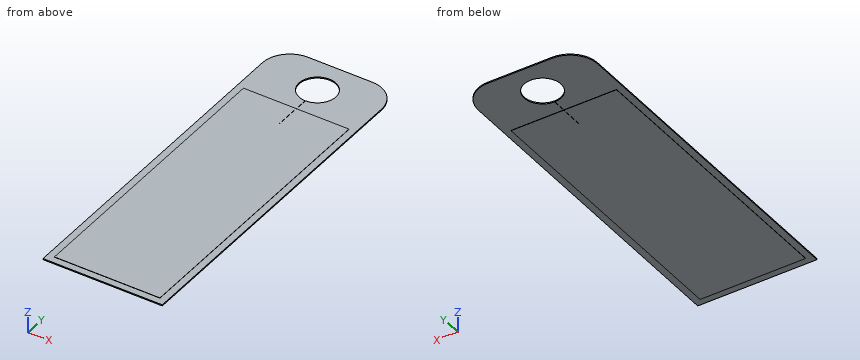
```python
from build123d import *

# Parameters (mm, degrees)
SKETCH2_R                = 8
BOSS_EXTRUDE1_DEPTH      = 0.5
BOSS_EXTRUDE2_DEPTH      = 0.1
BOSS_EXTRUDE2_DEPTH_BACK = 0.6
SKETCH4_W                = 46
SKETCH4_H                = 125
CUT_EXTRUDE1_DEPTH       = 145.361906333
CUT_EXTRUDE1_DEPTH_BACK  = 145.361906333
SKETCH5_W                = 0.1
SKETCH5_H                = 25


with BuildPart() as part:
    # Sketch2 → Boss-Extrude1 (new body)
    with BuildSketch(Plane.XY):
        with BuildLine():
            Line((-14, 15), (14, 15))
            ThreePointArc((14, 15), (22.485281374, 11.485281374), (26, 3))
            Line((26, 3), (26, -142))
            Line((26, -142), (-26, -142))
            Line((-26, -142), (-26, 3))
            ThreePointArc((-26, 3), (-22.485281374, 11.485281374), (-14, 15))
        make_face()
        Circle(SKETCH2_R, mode=Mode.SUBTRACT)
    extrude(amount=BOSS_EXTRUDE1_DEPTH)

    # Sketch4 → Boss-Extrude2 (add, two sides: drawn at the far end of the back side and taken through both)
    with BuildSketch(Plane.XY.offset(0.5).offset(-BOSS_EXTRUDE2_DEPTH_BACK)):
        with Locations((0, -76.5)):
            Rectangle(SKETCH4_W, SKETCH4_H)
    extrude(amount=BOSS_EXTRUDE2_DEPTH + BOSS_EXTRUDE2_DEPTH_BACK)

    # Sketch5 → Cut-Extrude1 (cut, two sides: drawn at the far end of the back side and taken through both)
    with BuildSketch(Plane.XY.offset(0.5).offset(-CUT_EXTRUDE1_DEPTH_BACK)):
        with Locations((0, -12.5)):
            Rectangle(SKETCH5_W, SKETCH5_H)
    extrude(amount=CUT_EXTRUDE1_DEPTH + CUT_EXTRUDE1_DEPTH_BACK, mode=Mode.SUBTRACT)


solid = part.part
```
Build history of the part. All positions in model axes, mm. Coordinates: 2 decimals unless noted, no trailing zeros. Write each loop counter-clockwise with the first axis right and the second up, starting at its lowest first coordinate (ties: lowest second). Pieces come first, ordered by that corner, then holes.
1. Band-saw the part on C-C, the plane x = 16. Give the cut face in (y, z).
Answer block:
outline: (-142, 0) - (-139, 0) - (-139, -0.1) - (-14, -0.1) - (-14, 0) - (14.83, 0) - (14.83, 0.5) - (-14, 0.5) - (-14, 0.6) - (-139, 0.6) - (-139, 0.5) - (-142, 0.5) - close
2. Band-saw the part on B-B, the plane y = -95. Give the cut face in (x, z), and give its area (3 significant figures).
Answer block:
outline: (-26, 0) - (-23, 0) - (-23, -0.1) - (23, -0.1) - (23, 0) - (26, 0) - (26, 0.5) - (23, 0.5) - (23, 0.6) - (-23, 0.6) - (-23, 0.5) - (-26, 0.5) - close
area: 35.2 mm2
3. Band-saw the part on A-A, the plane x = -3. Give the cut face in (y, z), and give its area (3 significant figures).
Answer block:
outline: (-142, 0) - (-139, 0) - (-139, -0.1) - (-14, -0.1) - (-14, 0) - (-7.42, 0) - (-7.42, 0.5) - (-14, 0.5) - (-14, 0.6) - (-139, 0.6) - (-139, 0.5) - (-142, 0.5) - close; (7.42, 0) - (15, 0) - (15, 0.5) - (7.42, 0.5) - close
area: 96.1 mm2
4. Drill centre lines: probe 1 along Y at (x, z) = (0, 0.3); probe 2 along X at (y, z) = (0, 0.2); probe 3 along Z at (x, y) = (23, -10). Where is each one in solid material? Low to high.
Answer block:
probe 1: y = -142 to -25, 8 to 15
probe 2: x = -26 to -8, 8 to 26
probe 3: z = 0 to 0.5
